Geometry: final body of the model. Coordinates: model frame, mm. Coordinates: 2 decimals unless noted, no trailing zeros. Loops run counter-clockwise (first coordinate to the right, second up) from the corner with the lowest first, then second, coordinate; pieces in that order, holes last. Notation, with made-up numbers: (74, 38) -> (79, 38) arc R12 cw to (79, 53) -> close; hole circle Ø9 at (-20, 27). An arc over 180 degrees is marked (long way). One line per item, written item: value. Start each with the question number.
from build123d import *

# Parameters (mm, degrees)
SKETCH1_R           = 32
SKETCH1_R_2         = 1.4732
SKETCH1_R_3         = 19
BOSS_EXTRUDE1_DEPTH = 3.175


with BuildPart() as part:
    # Sketch1 → Boss-Extrude1 (new body)
    with BuildSketch(Plane.XY.offset(0.2)):
        with Locations((-17.5, -28.25)):
            Circle(SKETCH1_R)
        with Locations((-17.5, -55.7)):
            Circle(SKETCH1_R_2, mode=Mode.SUBTRACT)
        with Locations((-31.225, -52.022397334)):
            Circle(SKETCH1_R_2, mode=Mode.SUBTRACT)
        with Locations((-41.272397334, -41.975)):
            Circle(SKETCH1_R_2, mode=Mode.SUBTRACT)
        with Locations((-44.95, -28.25)):
            Circle(SKETCH1_R_2, mode=Mode.SUBTRACT)
        with Locations((-41.272397334, -14.525)):
            Circle(SKETCH1_R_2, mode=Mode.SUBTRACT)
        with Locations((-31.225, -4.477602666)):
            Circle(SKETCH1_R_2, mode=Mode.SUBTRACT)
        with Locations((-17.5, -0.8)):
            Circle(SKETCH1_R_2, mode=Mode.SUBTRACT)
        with Locations((-3.775, -4.477602666)):
            Circle(SKETCH1_R_2, mode=Mode.SUBTRACT)
        with Locations((6.272397334, -14.525)):
            Circle(SKETCH1_R_2, mode=Mode.SUBTRACT)
        with Locations((9.95, -28.25)):
            Circle(SKETCH1_R_2, mode=Mode.SUBTRACT)
        with Locations((6.272397334, -41.975)):
            Circle(SKETCH1_R_2, mode=Mode.SUBTRACT)
        with Locations((-3.775, -52.022397334)):
            Circle(SKETCH1_R_2, mode=Mode.SUBTRACT)
        with Locations((-17.5, -28.25)):
            Circle(SKETCH1_R_3, mode=Mode.SUBTRACT)
    extrude(amount=BOSS_EXTRUDE1_DEPTH)


solid = part.part
1. Section B-B on x = -17.5. Return the cut outline in (y, z) (3 decimals).
2. Section A-A on y = -28.25. Return the cut outline in (x, z) (3 decimals).
3. Pin query (flat end, axial travel): pin 1 Ø1.5 at (y, z) = (-36.5, 1) entering from -X; pin 2 Ø2.5 at (x, y) = (9.95, -28.25) entering from -Z. Return the tip coordinate at first contact, or that it passes through.
4. Section C-C on z = 1.05. Count the separate pieces of the cut face and the enclosed holes in it, plus the area to 3 significant figures.
5. Line query: L1, parallel to Y at x = -17.5, z = 1.1; L2, parallel to Y at x = -2.5, z = 2.65; L3, parallel to Y at x = -40, z = 2.6. Output: solid intervals per line, ascending. Write a range as [from, to].
6. Section D-D on x = -44.95. Return the cut outline in (y, z) (3 decimals).
7. Draft query along X for faces 1 (the face through (-4, -42, 3.375)), 2 (the face through (-32.394, -5.374, 1.765)), 3 (the face through (-24.44, -59.49, 1.77)). Return one class per face: released by +X, released by -X, zero draft, split by the parting line, or undercut.
Checks:
1. outline: (-60.25, 0.2) -> (-57.173, 0.2) -> (-57.173, 3.375) -> (-60.25, 3.375) -> close; (-54.227, 0.2) -> (-47.25, 0.2) -> (-47.25, 3.375) -> (-54.227, 3.375) -> close; (-9.25, 0.2) -> (-2.273, 0.2) -> (-2.273, 3.375) -> (-9.25, 3.375) -> close; (0.673, 0.2) -> (3.75, 0.2) -> (3.75, 3.375) -> (0.673, 3.375) -> close
2. outline: (-49.5, 0.2) -> (-46.423, 0.2) -> (-46.423, 3.375) -> (-49.5, 3.375) -> close; (-43.477, 0.2) -> (-36.5, 0.2) -> (-36.5, 3.375) -> (-43.477, 3.375) -> close; (1.5, 0.2) -> (8.477, 0.2) -> (8.477, 3.375) -> (1.5, 3.375) -> close; (11.423, 0.2) -> (14.5, 0.2) -> (14.5, 3.375) -> (11.423, 3.375) -> close
3. pin 1: x = -48.61
3. pin 2: through
4. separate pieces: 1
4. enclosed holes: 13
4. area: 2,000 mm²
5. L1: [-60.25, -57.17], [-54.23, -47.25], [-9.25, -2.27], [0.67, 3.75]
5. L2: [-56.52, -52.76], [-51.28, -39.91], [-16.59, -5.22], [-3.74, 0.02]
5. L3: [-51, -42.72], [-41.23, -15.27], [-13.78, -5.5]
6. outline: (-44.697, 0.2) -> (-29.723, 0.2) -> (-29.723, 3.375) -> (-44.697, 3.375) -> close; (-26.777, 0.2) -> (-11.803, 0.2) -> (-11.803, 3.375) -> (-26.777, 3.375) -> close
7. face 1: zero draft
7. face 2: undercut
7. face 3: split by the parting line
